The model under review builds one solid part; all positions refer to its coordinate system, in mm. A direction names the side the tool comes from. Coordinates: 2 decimals unless noted, no trailing zeros. Order: outer loops, then holes, each group sorted by start corner. A loop starts at its lowest first (then second) coordinate and runs counter-clockwise, first axis right, second up. Notation, with made-up numbers: (30, -30) -> (41, -30) arc R8 cw to (41, -21) -> close; hole circle Ø5 at (52, -3). An arc over 180 degrees is marked (long way). Use one line per item in the form item = value. Start each with the question number.
(1) Take a section at D-D (x = 0.05). State the section outline as (y, z) points.
(2) Take a section at B-B (y = 7.5). State the section outline as (x, z) points.
(3) Take a section at C-C (y = -0.5). State the section outline as (x, z) points, then the cut area to 3 significant figures.
(4) Take a section at A-A (x = -1.28). State the section outline as (y, z) points.
(5) For faces 5 (the flat face through (0, 3.361, -0.5)), 6 (the flat face through (1.863, -0.6, -0.5)), 7 (the flat face through (0, 0.407, 2)), 8 (the flat face through (0, 3.893, 2)), list the 3-axis set-ups (+Z, -Z, +X, -X, +Y, -Y) from which the entire face can be reached by the end or side of a thin tool; tool diameter is ignored.
(6) Insertion check: pin 1 Ø0.6 at (x, y) = (-1.28, -6.19) entering from -Z; pin 2 Ø0.6 at (y, z) = (-2, -0.5) entering from -X; pin 3 Ø0.9 at (x, z) = (0, -0.5) entering from +Y; pin 4 Ø0.6 at (y, z) = (0.5, -0.5) entering from +X. Each pin has a flat end and moves straight along its axis. Give the tip position at first contact, or say it passes through.
(7) Mouldability with a two-part tool opening along Y and no side actions: class faces 1 (the flat face through (0, 2, 2.52)), 2 (the cylindrical face through (-1.39, -9.23, 0.5)), 3 (the cylindrical face through (1.17, -6.69, 0.5)), 4 (the flat face through (0, -4.546, -0.5)) as +Y half, -Y half, draft (parallel to the pull), parting line (faces both ways), or undercut.
(8) Wall thickness on line 1 along Y through (x, z) = (-1.28, 0.7); line 2 along Y through (x, z) = (0.85, 0.85); line 3 along Z through (x, y) = (0.2, 5.75): over which ranges is each line inside the solid? List them lowest first.
```python
from build123d import *

# Parameters (mm, degrees)
SKETCH1_W           = 5.1
SKETCH1_H           = 20
SKETCH1_R           = 1.09
SKETCH1_R_2         = 0.51
BOSS_EXTRUDE1_DEPTH = 1.02
SKETCH2_W           = 3.667230494
SKETCH2_H           = 3.486682144
BOSS_EXTRUDE2_DEPTH = 1.5
SKETCH3_W           = 3.726930802
SKETCH3_H           = 7.906409835
BOSS_EXTRUDE3_DEPTH = 1.1


with BuildPart() as part:
    # Sketch1 → Boss-Extrude1 (new body)
    with BuildSketch(Plane.XY):
        Rectangle(SKETCH1_W, SKETCH1_H)
        with Locations((0.05, 7.5)):
            Circle(SKETCH1_R, mode=Mode.SUBTRACT)
        with Locations((-1.28, -6.19)):
            Circle(SKETCH1_R_2, mode=Mode.SUBTRACT)
        with Locations((1.28, -6.19)):
            Circle(SKETCH1_R_2, mode=Mode.SUBTRACT)
        with Locations((1.28, -8.73)):
            Circle(SKETCH1_R_2, mode=Mode.SUBTRACT)
        with Locations((-1.28, -8.73)):
            Circle(SKETCH1_R_2, mode=Mode.SUBTRACT)
    extrude(amount=BOSS_EXTRUDE1_DEPTH)

    # Sketch2 → Boss-Extrude2 (add)
    with BuildSketch(Plane.XY.offset(1.02)):
        with Locations((0, 2.15)):
            Rectangle(SKETCH2_W, SKETCH2_H)
    extrude(amount=BOSS_EXTRUDE2_DEPTH)

    # Sketch3 → Boss-Extrude3 (add)
    with BuildSketch(Plane(origin=(0, 0, 0), x_dir=(-1, 0, 0), z_dir=(0, 0, -1))):
        with Locations((0, -0.592550596)):
            Rectangle(SKETCH3_W, SKETCH3_H)
    extrude(amount=BOSS_EXTRUDE3_DEPTH)


solid = part.part
```
Findings:
q1.outline = (-10, 0) -> (-4.55, 0) -> (-4.55, -1.1) -> (3.36, -1.1) -> (3.36, 0) -> (6.41, 0) -> (6.41, 1.02) -> (3.89, 1.02) -> (3.89, 2.52) -> (0.41, 2.52) -> (0.41, 1.02) -> (-10, 1.02) -> close; (8.59, 0) -> (10, 0) -> (10, 1.02) -> (8.59, 1.02) -> close
q2.outline = (-2.55, 0) -> (-1.04, 0) -> (-1.04, 1.02) -> (-2.55, 1.02) -> close; (1.14, 0) -> (2.55, 0) -> (2.55, 1.02) -> (1.14, 1.02) -> close
q3.outline = (-2.55, 0) -> (-1.86, 0) -> (-1.86, -1.1) -> (1.86, -1.1) -> (1.86, 0) -> (2.55, 0) -> (2.55, 1.02) -> (-2.55, 1.02) -> close
q3.area = 9.30 mm²
q4.outline = (-10, 0) -> (-9.24, 0) -> (-9.24, 1.02) -> (-10, 1.02) -> close; (-8.22, 0) -> (-6.7, 0) -> (-6.7, 1.02) -> (-8.22, 1.02) -> close; (-5.68, 0) -> (-4.55, 0) -> (-4.55, -1.1) -> (3.36, -1.1) -> (3.36, 0) -> (10, 0) -> (10, 1.02) -> (3.89, 1.02) -> (3.89, 2.52) -> (0.41, 2.52) -> (0.41, 1.02) -> (-5.68, 1.02) -> close
q5.face_5 = -Z, +X, -X, +Y
q5.face_6 = -Z, +X, +Y, -Y
q5.face_7 = +Z, +X, -X, -Y
q5.face_8 = +Z, +X, -X, +Y
q6.pin_1 = through
q6.pin_2 = -1.86
q6.pin_3 = 3.36
q6.pin_4 = 1.86
q7.face_1 = draft
q7.face_2 = undercut
q7.face_3 = undercut
q7.face_4 = -Y half
q8.line_1 = -10 to -9.24, -8.22 to -6.7, -5.68 to 10
q8.line_2 = -10 to -9, -8.46 to -6.46, -5.92 to 6.76, 8.24 to 10
q8.line_3 = 0 to 1.02
